The drawing under review shows one solid part. Ordinate dimensions are in mm from its lowest x, y, z. Round coordinates to 2 decimals unless told otherwise and drop trailing zeros. Write each loop counter-clockwise with the first axis right and the second up, starting at its lowest first coordinate (ties: lowest second). Pieces come first, ordered by that corner, then holes. Notation, with made-up numbers: (-11, 88.25) -> (44, 88.25) arc R17 cw to (44, 111.25) -> close; hole circle Ø9 at (33.5, 5). An arc over 180 degrees is marked (long way). Answer in a Markdown table with one row per item. Add a question column.
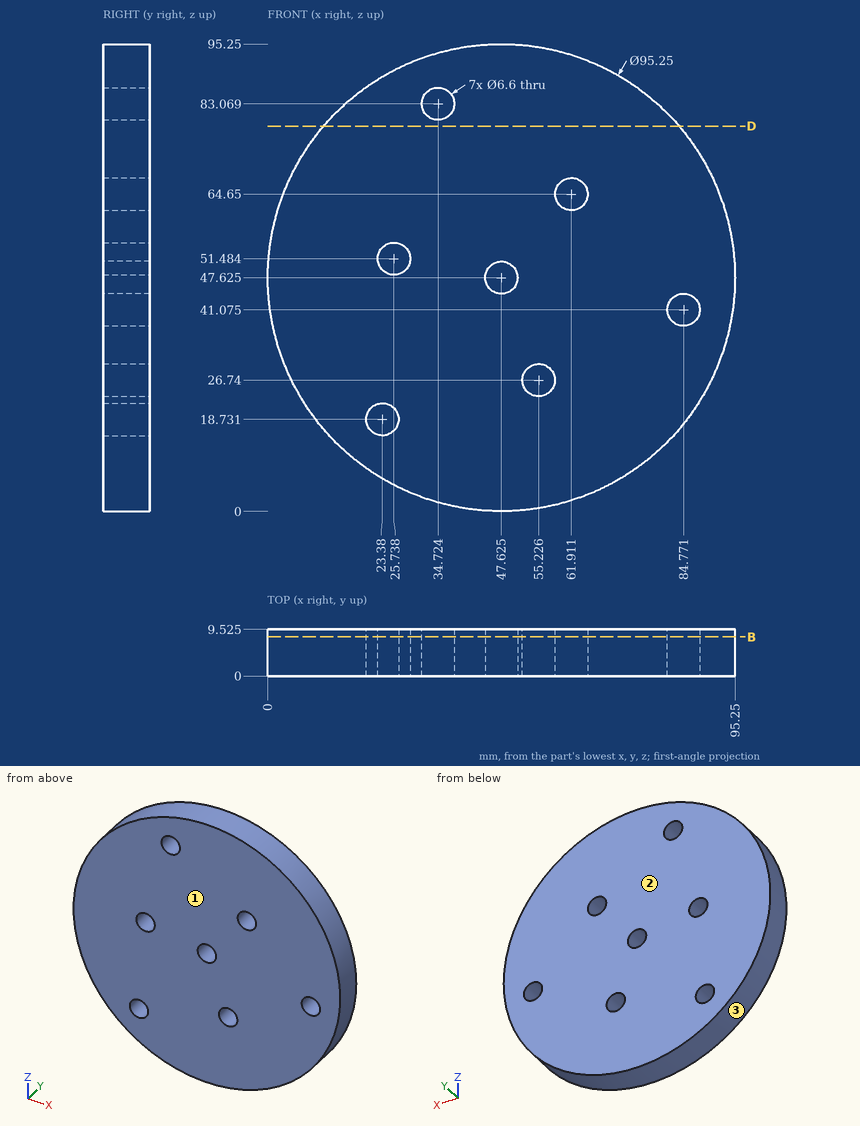
1. For L1, parallel to X at y = 7.25, z = 48; L2, parallel to Z at x = 63.5, y = 8 (1 decimal); L3, parallel to X at y = 3.5, z = 82 (1 decimal), list the stretches that pass through material, from the lowest coordinate up.
2. Mouldability with a two-part tool opening along Y and no side actions: class the marked faces 1, 2 and 3 as pulls with the +Y half, pulls with the -Y half, needs draft (parallel to the pull), parting line crosses it, or undercut.
3. Add section D-D on z = 78.5. Write out the cut boundary in (x, y) (1 decimal), plus the area to 3 significant figures.
4. Insertion check: pin 1 Ø4 at (x, z) = (25.74, 51.48) entering from -Y; pin 2 Ø5 at (x, y) = (47.5, 2) entering from -Z; pin 3 Ø4 at (x, y) = (73, 4.5) entering from -Z. Each pin has a flat end and moves straight along its axis. Give the tip position at first contact, or say it passes through.
5. Add section B-B on y = 8. State how many separate pieces and enclosed holes the cut face has, plus the area to 3 significant figures.
Filled in:
| question | item | result |
|---|---|---|
| 1 | L1 | 0 to 44.35, 50.9 to 95.25 |
| 1 | L2 | 2.7 to 61.8, 67.5 to 92.5 |
| 1 | L3 | 14.7 to 31.6, 37.8 to 80.6 |
| 2 | face 1 | pulls with the -Y half |
| 2 | face 2 | pulls with the +Y half |
| 2 | face 3 | needs draft |
| 3 | outline | (11.4, 0) -> (83.9, 0) -> (83.9, 9.5) -> (11.4, 9.5) -> close |
| 3 | area | 691 mm² |
| 4 | pin 1 | through |
| 4 | pin 2 | z = 0 |
| 4 | pin 3 | z = 6.13 |
| 5 | separate pieces | 1 |
| 5 | enclosed holes | 7 |
| 5 | area | 6,890 mm² |
